Job drawing, mm, ordinate dimensions from the low corner. One solid piece. Give positions to 0.01 mm unless a question says otherwise; leave off trailing zeros. Order: outer loops, then holes, each group sorted by start corner. A loop starts at its lowest first (then second) coordinate and runs counter-clockwise, first axis right, second up. Notation, with made-up numbers: (-19, -4.75) - (2, -4.75) arc R34 ccw to (2, 28.25) - close; hole circle Ø4 at (-13.75, 37). An arc over 180 degrees is marked (long way). Use one line per item in the form item = value. Start each with the question number.
1. Drill centre lines: line 1 (Y direction, x = 31.5, z = 19); line 2 (X direction, y = 7, z = 34.5) (1 decimal); line 3 (Z direction, x = 32.5, y = 18.5) (1 decimal). Where is each one in solid material? Low to high.
2. Pull direction X, two halves, no side cores. Call the marked faces 1, 2, 3 and 4: +X half, -X half, draft (parallel to the pull), parting line (faces both ways), or undercut.
3. Band-saw the part on B-B, the plane x = 37. List the corners of the cut face in (y, z) (1 decimal), plus the area to 3 significant figures.
4. Pin check, flat tip, straight feed: P1, Ø19.5, axis at x = 26.5, z = 25, coming from the -Y side. Stop position of the tip, or through.
5. Band-saw the part on A-A, the plane z = 16. List the corners of the cut face in (x, y), plus the area to 3 significant figures.
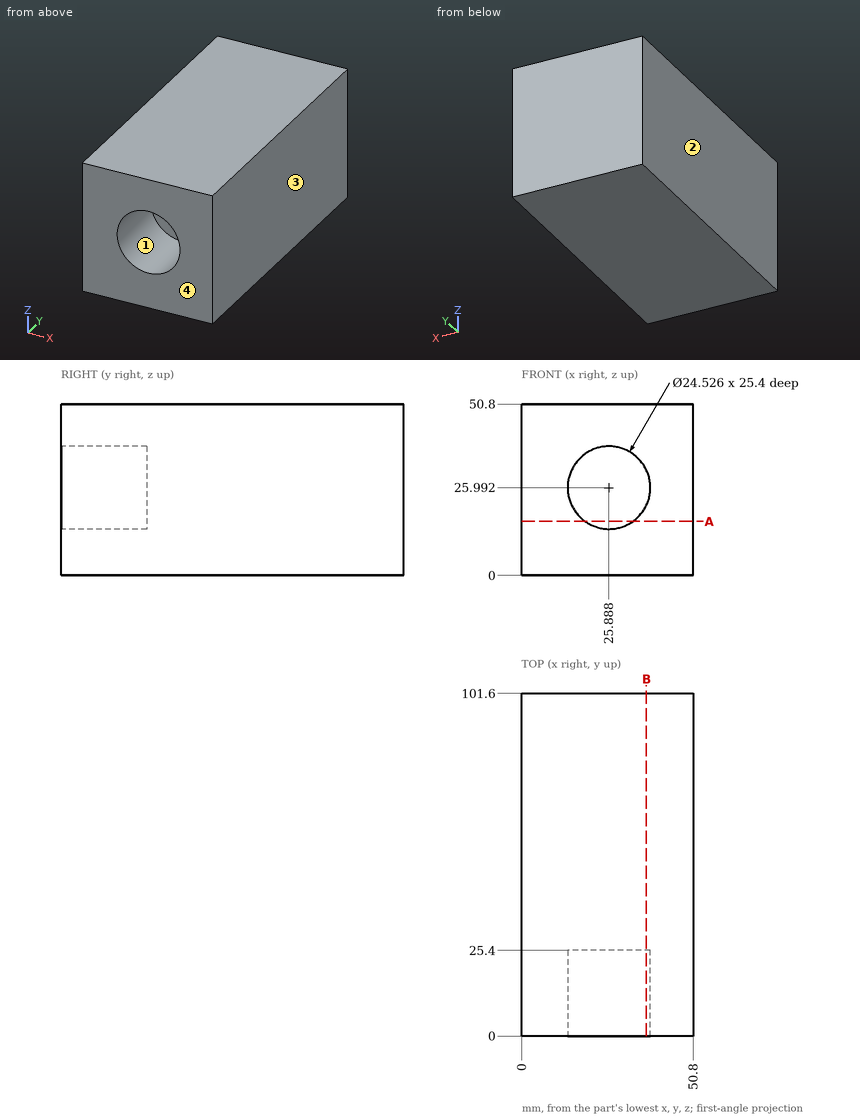
From the geometry:
q1.line_1 = 25.4 to 101.6
q1.line_2 = 0 to 17.1, 34.7 to 50.8
q1.line_3 = 0 to 15.7, 36.3 to 50.8
q2.face_1 = undercut
q2.face_2 = -X half
q2.face_3 = +X half
q2.face_4 = draft
q3.outline = (0, 0) - (101.6, 0) - (101.6, 50.8) - (0, 50.8) - (0, 31.2) - (25.4, 31.2) - (25.4, 20.8) - (0, 20.8) - close
q3.area = 4,900 mm²
q4.P1 = 25.4
q5.outline = (0, 0) - (18.78, 0) - (18.78, 25.4) - (33, 25.4) - (33, 0) - (50.8, 0) - (50.8, 101.6) - (0, 101.6) - close
q5.area = 4,800 mm²
